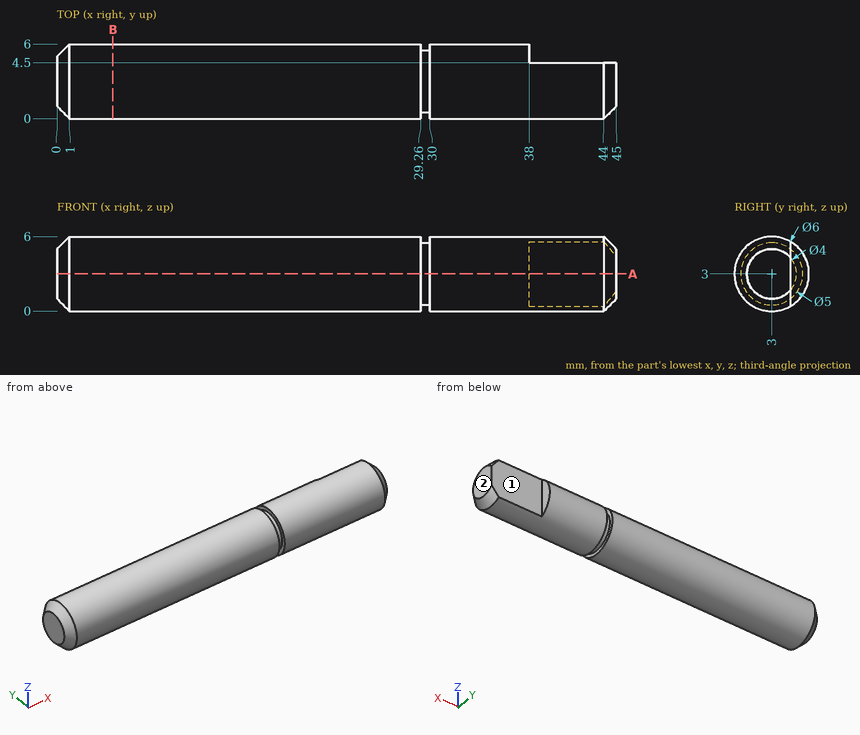
Geometry check sheet. Reference: drawing and pictorial views, mm from the part's lowest x, y, z. A direction names the side the tool comes from. Give positions to 0.01 mm unless a question says otherwise; leave off trailing zeros. Order: outer loops, then holes, each group sorted by start corner. A loop starts at its lowest first (then second) coordinate and runs counter-clockwise, first axis right, second up. Notation, with made-up numbers: M 32.25,-26 L 59.25,-26 A24 cw 59.25,9 Z; hole C 32.25,-6.5 d9. An arc over 180 degrees is marked long. Answer in a Markdown table with one row per item. Add a question column.
Item 1: Gauge pin test, flat ends, axial feed: pin 1 (0.8 mm diameter, centred on y = 5, z = 3, fed in from +X); pin 2 (1.6 mm diameter, centred on x = 42.5, z = 2, fed in from +Y); pin 3 (1.5 mm diameter, centred on x = 25.5, y = 2, fed in from +Z); pin 4 (3 mm diameter, centred on y = 3.5, z = 3.5, fed in from -X). Record the tip position at first contact, or that the pin passes through.
Item 2: Tool access check on the marked faces 1 and 2. Record the directions out of +Z, -Z, +X, -X, +Y, -Y that give a thin tool (end or side, any length) a straight path to the whole face; none if there is none.
Item 3: Scan lines: probe 1 along Z at (x, y) = (7.5, 3.15); probe 2 along Z at (x, y) = (17.5, 0.6); probe 3 along Y at (x, z) = (17.5, 1.75). Record each from-to range of solid material in increasing order. Write a range as from..to.
Item 4: Section check A-A, the plane z = 3. Enter the section's corners in (x, y), and give its area (3 significant figures).
Item 5: Section check B-B, the plane x = 4.5. Enter the section's corners in (y, z).
Filled sheet:
| question | item | result |
|---|---|---|
| 1 | pin 1 | stops at x = 38 |
| 1 | pin 2 | stops at y = 4.5 |
| 1 | pin 3 | stops at z = 5.99 |
| 1 | pin 4 | stops at x = 0 |
| 2 | face 1 | +Z, -Z, +X, +Y |
| 2 | face 2 | +Z, -Z, +X, +Y, -Y |
| 3 | probe 1 | z = 0..6 |
| 3 | probe 2 | z = 1.2..4.8 |
| 3 | probe 3 | y = 0.27..5.73 |
| 4 | outline | M 0,1 L 1,0 L 29.26,0 L 29.26,0.5 L 30,0.5 L 30,0 L 44,0 L 45,1 L 45,4.5 L 38,4.5 L 38,6 L 30,6 L 30,5.5 L 29.26,5.5 L 29.26,6 L 1,6 L 0,5 Z |
| 4 | area | 257 mm^2 |
| 5 | outline | C 3,3 d6 |
